from build123d import *

# Parameters (mm, degrees)
F0_W     = 27.432
F0_H     = 32.512
F1_DEPTH = 27.3
F0_H_2   = 8.89
F2_DEPTH = 2.2
F3_SIZE  = 2.5
F4_W     = 14.732
F4_H     = 11.212
F5_DEPTH = 7.3
F6_W     = 8.5
F6_H     = 5.3
F6_W_2   = 5.6
F6_H_2   = 10.3
F6_W_3   = 10.5
F6_H_3   = 5.6
F7_DEPTH = 7.3
F9_DEPTH = 27.301


with BuildPart() as f1:
    # F0 (on Top) → F1 (new body)
    with BuildSketch(Plane.XY):
        Rectangle(F0_W, F0_H)
    extrude(amount=F1_DEPTH)

    # F0 (on Top) → F2 (join)
    with BuildSketch(Plane.XY):
        with Locations((0, 20.701)):
            Rectangle(F0_W, F0_H_2)
        with Locations((0, -20.701)):
            Rectangle(F0_W, F0_H_2)
    extrude(amount=F2_DEPTH)

    # F3
    f3_edges = [f1.edges().sort_by_distance(p)[0] for p in [
        (-13.716, -25.146, 1.1),
        (13.716, -25.146, 1.1),
        (13.716, 25.146, 1.1),
        (-13.716, 25.146, 1.1),
    ]]
    chamfer(f3_edges, length=F3_SIZE)

    # F4 (on face) → F5 (cut)
    with BuildSketch(Plane.XY.offset(27.3)):
        with Locations((6.35, -10.65)):
            Rectangle(F4_W, F4_H)
        Polygon((-13.716, 16.256), (-13.716, -1.106), (5.916, -1.106), (5.916, 5.294), (-7.784, 5.294), (-7.784, 16.256), align=None)
    extrude(amount=-F5_DEPTH, mode=Mode.SUBTRACT)

    # F6 (on face) → F7 (cut)
    with BuildSketch(Plane.XY.offset(27.3)):
        with Locations((-2.034, 11.706)):
            Rectangle(F6_W, F6_H)
        with Locations((8.266, 11.706)):
            Rectangle(F6_W, F6_H)
        with Locations((10.166, 2.106)):
            Rectangle(F6_W_2, F6_H_2)
        with Locations((-7.716, -12.706)):
            Rectangle(F6_W_3, F6_H_3)
        with Locations((-7.716, -5.256)):
            Rectangle(F6_W_3, F6_H_3)
    extrude(amount=-F7_DEPTH, mode=Mode.SUBTRACT)

    # F8 (on face) → F9 (cut, through all)
    with BuildSketch(Plane.XY):
        with BuildLine():
            Line((-1.8, -25.146), (0, -25.146))
            Line((0, -25.146), (1.8, -25.146))
            Line((1.8, -25.146), (1.8, -21.8))
            ThreePointArc((1.8, -21.8), (1.272792, -20.527208), (0, -20))
            ThreePointArc((0, -20), (-1.272792, -20.527208), (-1.8, -21.8))
            Line((-1.8, -21.8), (-1.8, -25.146))
        make_face()
        with BuildLine():
            Line((1.8, 25.146), (0, 25.146))
            Line((0, 25.146), (-1.8, 25.146))
            Line((-1.8, 25.146), (-1.8, 21.8))
            ThreePointArc((-1.8, 21.8), (-1.272792, 20.527208), (0, 20))
            ThreePointArc((0, 20), (1.272792, 20.527208), (1.8, 21.8))
            Line((1.8, 21.8), (1.8, 25.146))
        make_face()
    extrude(amount=F9_DEPTH, mode=Mode.SUBTRACT)


solid = f1.part
Could you check a few things on this model? Use its own coordinates, in mm. A direction names the side the tool comes from. Give positions to 0.01 mm unless a question says otherwise; leave off trailing zeros. Order: outer loops, then holes, each group sorted by start corner. A loop starts at its lowest first (then second) coordinate and runs counter-clockwise, first axis right, second up.
1. For pin 1 (1 mm diameter, centred on x = -0.5, y = 2.5, fed in from +Z); pin 2 (1.5 mm diameter, centred on x = 10, y = 17, fed in from -Z); pin 3 (5 mm diameter, centred on x = 2, z = 16.5, fed in from -Y); pin 4 (0.7 mm diameter, centred on y = 23.5, z = 1, fed in from +X), each with a flat end and sliding along its axis, tell me the tip position at first contact or that it passes through.
Answers below:
pin 1: stops at z = 20
pin 2: stops at z = 0
pin 3: stops at y = -16.26
pin 4: stops at x = 13.21
2. I need wall thicknesses on L1, parallel to Y at x = -6.25, z = 26; L2, parallel to Y at x = 4.5, z = 23; L3, parallel to Y at x = 9.25, z = 22. Which ranges of each line are inside material? Lowest first, please.
Answers below:
L1: y = -16.26 to -15.51, -9.91 to -8.06, -2.46 to -1.11, 5.29 to 9.06, 14.36 to 16.26
L2: y = -5.04 to -1.11, 5.29 to 9.06, 14.36 to 16.26
L3: y = -5.04 to -3.04, 7.26 to 9.06, 14.36 to 16.26
3. Thinking about a two-plate mould opening in X: for faces 4 (the flat face through (-8, -5, 20)), 5 (the flat face through (12.45, 23.91, 1.08)), 6 (the flat face through (1, -2, 27.3)), which applies, +X half, -X half, draft (parallel to the pull), parting line (faces both ways), or undercut?
Answers below:
face 4: undercut
face 5: +X half
face 6: draft
4. Suppose I cut it at C-C (y = 13). Write out the boundary of the cut face in (x, z), plus the area to 3 significant figures.
Answers below:
outline: (-13.72, 0) - (13.72, 0) - (13.72, 27.3) - (12.52, 27.3) - (12.52, 20) - (4.02, 20) - (4.02, 27.3) - (2.22, 27.3) - (2.22, 20) - (-6.28, 20) - (-6.28, 27.3) - (-7.78, 27.3) - (-7.78, 20) - (-13.72, 20) - close
area: 581 mm2
5. Which directions (+Z, -Z, +X, -X, +Y, -Y) give clear straight access to the entire face, cutting with the end or side of a thin tool? Please do faces 1 (the flat face through (1.8, -23, 1)), 2 (the flat face through (-7, 25.146, 1)), 3 (the flat face through (10, 2, 20)).
Answers below:
face 1: +Z, -Z, -Y
face 2: +Z, -Z, +X, -X, +Y
face 3: +Z
6. Suppose I cut it at A-A (y = -0.5). Write out the boundary of the cut face in (x, z), plus the area to 3 significant figures.
Answers below:
outline: (-13.72, 0) - (13.72, 0) - (13.72, 27.3) - (12.97, 27.3) - (12.97, 20) - (7.37, 20) - (7.37, 27.3) - (5.92, 27.3) - (5.92, 20) - (-13.72, 20) - close
area: 565 mm2
7. Suppose I cut it at D-D (z = 4.5). Write out the boundary of the cut face in (x, y), plus the area to 3 significant figures.
Answers below:
outline: (-13.72, -16.26) - (13.72, -16.26) - (13.72, 16.26) - (-13.72, 16.26) - close
area: 892 mm2
8. Suppose I cut it at B-B (x = 3.5). Write out the boundary of the cut face in (y, z), plus the area to 3 significant figures.
Answers below:
outline: (-25.15, 0) - (25.15, 0) - (25.15, 2.2) - (16.26, 2.2) - (16.26, 27.3) - (5.29, 27.3) - (5.29, 20) - (-1.11, 20) - (-1.11, 27.3) - (-5.04, 27.3) - (-5.04, 20) - (-16.26, 20) - (-16.26, 2.2) - (-25.15, 2.2) - close
area: 798 mm2
